Input: part model. Units: mm. Frame: model coordinates. A direction names the side the tool comes from. Coordinates: 2 decimals unless noted, no trailing zeros. Order: outer loops, then holes, each group sorted by start corner. A loop starts at its lowest first (then second) coordinate and runs counter-clockwise, first axis right, second up. Notation, with made-up numbers: (38, 25.25) - (46, 25.25) arc R15 cw to (46, 50.25) - close; hole circle Ø4 at (29.25, 35.5). An arc over 180 degrees is marked (long way). Answer as CSV lines item,"result". Start each with the question number.
Item 1: Access query for faces 5 (the flat face through (-2.286, 71, -34)), 6 (the cylindrical face through (-1.13, 11.27, 22.31)). Directions: +Z, -Z, +X, -X, +Y, -Y. A direction counts if a zero-diameter tool reaches every point of the face in a straight line with its end or side. Return the directions, or none.
Item 2: First-contact query: pin 1 (10.5 mm diameter, centred on y = 11.13, z = 19.05, fed in from -X); pin 2 (5 mm diameter, centred on x = -3.5, y = 38.5, fed in from -Z); pin 3 (6 mm diameter, centred on x = -4.5, z = -79, fed in from -Y). Flat tips, straight axial feed; report the tip coordinate or a pass-through.
Item 3: Draft query along Z for faces 1 (the cylindrical face through (-13.85, 122.87, 10.29)), 2 (the flat face through (-1.13, 53.22, -84.97)), 3 (the flat face through (-2, 68, 31.75)), 4 (the cylindrical face through (-1.13, 12.11, -22.16)). Return one class per face: +Z half, -Z half, draft (parallel to the pull), parting line (faces both ways), or undercut.
Item 4: Section D-D (x = -12). State how many separate pieces and enclosed holes the cut face has, and give its area (3 significant figures).
Item 5: Material intervals for line 1 along X through (y, z) = (41.5, -23); line 2 along Y through (x, z) = (-1.65, -19.05); line 3 along Y through (x, z) = (-1.3, -19.05), sorted ascending.
Item 6: Section C-C (y = 78.5). Output: boundary loops of the cut face in (x, z), and give its area (3 significant figures).
from build123d import *

# Parameters (mm, degrees)
BASE_FLANGE1_DEPTH         = 2.286
CUT_EXTRUDE1_REACH         = 196.797
SKETCH4_R                  = 3.2639
SKETCH4_R_2                = 3.5687
SKETCHED_START             = 119.049056405
SKETCHED_BEND2_OUTLINE_R   = 3.5687
SKETCHED_BEND2_DEPTH       = 4.950943595
SKETCHED_START_2           = -139.7
SKETCHED_BEND2_2_DEPTH     = 171.45
SKETCHED_BEND2_3_DEPTH     = 171.45
SKETCHED_START_3           = 104.381009176
SKETCHED_BEND2_4_OUTLINE_R = 3.5687
SKETCHED_BEND2_4_DEPTH     = 2.286


with BuildPart() as part:
    # Base-Flange1: sheet metal written as solids
    # Sketch2 → Base-Flange1 (new body)
    with BuildSketch(Plane(origin=(0, 0, 0), x_dir=(0, 0, -1), z_dir=(1, 0, 0))):
        Polygon((-31.75, 0), (31.75, 0), (139.7, 107.95), (139.7, 135.7376), (-31.75, 135.7376), align=None)
    extrude(amount=-BASE_FLANGE1_DEPTH)

    # Sketch4 → Cut-Extrude1 (cut, up to next)
    with BuildSketch(Plane(origin=(0, 0, 0), x_dir=(0, 0, -1), z_dir=(1, 0, 0)), mode=Mode.PRIVATE) as cut_extrude1_sk1:
        with Locations((19.05, 11.1252)):
            Circle(SKETCH4_R)
    cut_extrude1_tool1 = extrude(cut_extrude1_sk1.sketch, amount=-CUT_EXTRUDE1_REACH, mode=Mode.PRIVATE) & part.part
    # Sketch4 → Cut-Extrude1 (cut, up to next)
    with BuildSketch(Plane(origin=(0, 0, 0), x_dir=(0, 0, -1), z_dir=(1, 0, 0)), mode=Mode.PRIVATE) as cut_extrude1_sk2:
        with Locations((-19.05, 11.1252)):
            Circle(SKETCH4_R)
    cut_extrude1_tool2 = extrude(cut_extrude1_sk2.sketch, amount=-CUT_EXTRUDE1_REACH, mode=Mode.PRIVATE) & part.part
    # Sketch4 → Cut-Extrude1 (cut, up to next)
    with BuildSketch(Plane(origin=(0, 0, 0), x_dir=(0, 0, -1), z_dir=(1, 0, 0)), mode=Mode.PRIVATE) as cut_extrude1_sk3:
        with Locations((-12.7, 127.7874)):
            Circle(SKETCH4_R_2)
    cut_extrude1_tool3 = extrude(cut_extrude1_sk3.sketch, amount=-CUT_EXTRUDE1_REACH, mode=Mode.PRIVATE) & part.part
    # Sketch4 → Cut-Extrude1 (cut, up to next)
    with BuildSketch(Plane(origin=(0, 0, 0), x_dir=(0, 0, -1), z_dir=(1, 0, 0)), mode=Mode.PRIVATE) as cut_extrude1_sk4:
        with Locations((120.65, 127.7874)):
            Circle(SKETCH4_R_2)
    cut_extrude1_tool4 = extrude(cut_extrude1_sk4.sketch, amount=-CUT_EXTRUDE1_REACH, mode=Mode.PRIVATE) & part.part
    add(cut_extrude1_tool1.solids().sort_by_distance((0, 11.1252, -19.05))[0], mode=Mode.SUBTRACT)
    add(cut_extrude1_tool2.solids().sort_by_distance((0, 11.1252, 19.05))[0], mode=Mode.SUBTRACT)
    add(cut_extrude1_tool3.solids().sort_by_distance((0, 127.7874, 12.7))[0], mode=Mode.SUBTRACT)
    add(cut_extrude1_tool4.solids().sort_by_distance((0, 127.7874, -120.65))[0], mode=Mode.SUBTRACT)

    # Sketched Bend2: read off the stored shape, not the designer's step
    # Sketched Bend2 outline → Sketched Bend2 (cut)
    with BuildSketch(Plane(origin=(0, 0, 0), x_dir=(0.906307787036651, -0.42261826174069705, 0), z_dir=(0.42261826174069705, 0.9063077870366512, 0)).offset(SKETCHED_START)):
        with Locations((-61.845865858, -12.7)):
            Circle(SKETCHED_BEND2_OUTLINE_R)
        with Locations((-61.845865858, 120.65)):
            Circle(SKETCHED_BEND2_OUTLINE_R)
    extrude(amount=SKETCHED_BEND2_DEPTH, mode=Mode.SUBTRACT)

    # Sketched Bend2 2 outline → Sketched Bend2 2 (cut)
    with BuildSketch(Plane.XY.offset(SKETCHED_START_2)):
        with BuildLine():
            Line((-2.286, 135.7376), (-2.286, 118.759838882))
            ThreePointArc((-2.286, 118.759838882), (-0.619280932, 117.279080961), (0, 115.137332236))
            Line((0, 115.137332236), (0, 135.7376))
            Line((0, 135.7376), (-2.286, 135.7376))
        make_face()
    extrude(amount=SKETCHED_BEND2_2_DEPTH, mode=Mode.SUBTRACT)

    # Sketched Bend2 3 outline → Sketched Bend2 3 (add)
    with BuildSketch(Plane.XY.offset(SKETCHED_START_2)):
        with BuildLine():
            Line((-19.143397335, 124.098413464), (-3.283253738, 116.702707046))
            ThreePointArc((-3.283253738, 116.702707046), (-2.556494295, 116.065356119), (-2.286, 115.137332236))
            Line((-2.286, 115.137332236), (-2.286, 118.759838882))
            ThreePointArc((-2.286, 118.759838882), (-2.301558441, 118.767216176), (-2.317148392, 118.774526647))
            Line((-2.317148392, 118.774526647), (-18.177291988, 126.170233065))
            Line((-18.177291988, 126.170233065), (-19.143397335, 124.098413464))
        make_face()
    extrude(amount=SKETCHED_BEND2_3_DEPTH)

    # Sketched Bend2 4 outline → Sketched Bend2 4 (cut)
    with BuildSketch(Plane(origin=(0, 0, 0), x_dir=(0.906307787036651, -0.42261826174069705, 0), z_dir=(0.42261826174069705, 0.9063077870366512, 0)).offset(SKETCHED_START_3)):
        with Locations((-61.845865858, -12.7)):
            Circle(SKETCHED_BEND2_4_OUTLINE_R)
        with Locations((-61.845865858, 120.65)):
            Circle(SKETCHED_BEND2_4_OUTLINE_R)
    extrude(amount=SKETCHED_BEND2_4_DEPTH, mode=Mode.SUBTRACT)


solid = part.part
Determined:
1,face 5,"+Z, -Z, -X, -Y"
1,face 6,"+X, -X"
2,pin 1,"stops at x = -2.29"
2,pin 2,"stops at z = -72.44"
2,pin 3,"stops at y = 45.23"
3,face 1,"undercut"
3,face 2,"-Z half"
3,face 3,"+Z half"
3,face 4,"undercut"
4,separate pieces,"3"
4,enclosed holes,"0"
4,area,"397 mm^2"
5,line 1,"x = -2.29 to 0"
5,line 2,"y = 0 to 7.86, 14.39 to 118.38"
5,line 3,"y = 0 to 7.86, 14.39 to 118.09"
6,outline,"(-2.29, -110.25) - (0, -110.25) - (0, 31.75) - (-2.29, 31.75) - close"
6,area,"325 mm^2"
